Autodesk Inventor part; units mm, degrees
ref_plane "YZ Plane" through (0, 0, 0) normal (1, 0, 0) x (0, 1, 0)
ref_plane "XZ Plane" through (0, 0, 0) normal (0, 1, 0) x (-1, 0, 0)
ref_plane "XY Plane" through (0, 0, 0) normal (0, 0, 1) x (1, 0, 0)
sketch "Эскиз1" plane through (0, 0, 0) normal (0, 0, 1) x (1, 0, 0)
  line L0 (0, 34.036) -> (-10.16, 44.196) construction
  line L1 (0, 0) -> (0, 34.036) construction
  line L2 (-10.16, -10.16) -> (0, 0) construction
  line L3 (-44.196, -10.16) -> (-10.16, -10.16) construction
  line L4 (-54.356, 0) -> (-44.196, -10.16) construction
  line L5 (-54.356, 34.036) -> (-54.356, 0) construction
  line L6 (-44.196, 44.196) -> (-54.356, 34.036) construction
  line L7 (-10.16, 44.196) -> (-44.196, 44.196) construction
  line L8 (1.5, -0.6213) -> (1.5, 34.6573)
  line L9 (1.5, 34.6573) -> (-9.5387, 45.696)
  line L10 (-9.5387, 45.696) -> (-44.8173, 45.696)
  line L11 (-44.8173, 45.696) -> (-55.856, 34.6573)
  line L12 (-55.856, 34.6573) -> (-55.856, -0.6213)
  line L13 (-55.856, -0.6213) -> (-44.8173, -11.66)
  line L14 (-44.8173, -11.66) -> (-9.5387, -11.66)
  line L15 (-9.5387, -11.66) -> (1.5, -0.6213)
  line L16 (-2.7356, -0.7983) -> (-25.2842, -0.7983) construction
  line L17 (-2.7356, 34.7503) -> (-2.7356, -0.7983) construction
  line L18 (-25.2842, 34.7503) -> (-2.7356, 34.7503) construction
  line L19 (-25.2842, -0.7983) -> (-25.2842, 34.7503) construction
  line L20 (-35.7877, 37.522) -> (-26.3913, 37.522) construction
  line L21 (-35.7877, -8.198) -> (-26.3913, -8.198) construction
  line L22 (-26.3913, -0.578) -> (-26.3913, -5.658) construction
  line L23 (-37.7413, -0.578) -> (-37.7413, -5.658) construction
  line L24 (-1.7356, -1.7983) -> (-26.2842, -1.7983)
  line L25 (-26.2842, -1.7983) -> (-26.2842, 35.7503)
  line L26 (-26.2842, 35.7503) -> (-1.7356, 35.7503)
  line L27 (-1.7356, 35.7503) -> (-1.7356, -1.7983)
  line L28 (-26.3913, 37.522) -> (-37.7413, 37.522) construction
  line L29 (-37.7413, 37.522) -> (-37.7413, -8.198) construction
  line L30 (-37.7413, -8.198) -> (-26.3913, -8.198) construction
  line L31 (-26.3913, -8.198) -> (-26.3913, 37.522) construction
  line L32 (-38.2413, 38.022) -> (-25.8913, 38.022)
  line L33 (-25.8913, 38.022) -> (-25.8913, -8.698)
  line L34 (-25.8913, -8.698) -> (-38.2413, -8.698)
  line L35 (-38.2413, -8.698) -> (-38.2413, 38.022)
  point P0 (-25.8913, -1.7983)
  point P1 (-25.8913, 35.7503)
  dimension "d0" = 1.5
  dimension "d1" = 1
  dimension "d2" = 0.5
extrude "Выдавливание1" add sketch "Эскиз1" along normal blind 2
sketch "Эскиз2" plane through (0, 0, 0) normal (0, 0, -1) x (-1, 0, 0)
  line L0 (-1.5, 34.6573) -> (9.5387, 45.696) construction
  line L1 (-1.5, -0.6213) -> (-1.5, 34.6573) construction
  line L2 (9.5387, -11.66) -> (-1.5, -0.6213) construction
  line L3 (44.8173, -11.66) -> (9.5387, -11.66) construction
  line L4 (55.856, -0.6213) -> (44.8173, -11.66) construction
  line L5 (55.856, 34.6573) -> (55.856, -0.6213) construction
  line L6 (44.8173, 45.696) -> (55.856, 34.6573) construction
  line L7 (9.5387, 45.696) -> (44.8173, 45.696) construction
  line L8 (1.7356, 35.7503) -> (1.7356, -1.7983) construction
  line L9 (25.8913, 35.7503) -> (1.7356, 35.7503) construction
  line L10 (25.8913, 38.022) -> (25.8913, 35.7503) construction
  line L11 (38.2413, 38.022) -> (25.8913, 38.022) construction
  line L12 (38.2413, -8.698) -> (38.2413, 38.022) construction
  line L13 (25.8913, -8.698) -> (38.2413, -8.698) construction
  line L14 (25.8913, -1.7983) -> (25.8913, -8.698) construction
  line L15 (1.7356, -1.7983) -> (25.8913, -1.7983) construction
  line L16 (-0.5, 34.2431) -> (9.9529, 44.696)
  line L17 (9.9529, 44.696) -> (44.4031, 44.696)
  line L18 (44.4031, 44.696) -> (54.856, 34.2431)
  line L19 (54.856, 34.2431) -> (54.856, -0.2071)
  line L20 (54.856, -0.2071) -> (44.4031, -10.66)
  line L21 (44.4031, -10.66) -> (9.9529, -10.66)
  line L22 (9.9529, -10.66) -> (-0.5, -0.2071)
  line L23 (-0.5, -0.2071) -> (-0.5, 34.2431)
  line L24 (-1.5, 34.6573) -> (9.5387, 45.696)
  line L25 (9.5387, 45.696) -> (44.8173, 45.696)
  line L26 (44.8173, 45.696) -> (55.856, 34.6573)
  line L27 (55.856, 34.6573) -> (55.856, -0.6213)
  line L28 (55.856, -0.6213) -> (44.8173, -11.66)
  line L29 (44.8173, -11.66) -> (9.5387, -11.66)
  line L30 (9.5387, -11.66) -> (-1.5, -0.6213)
  line L31 (-1.5, -0.6213) -> (-1.5, 34.6573)
  point P0 (0, 0)
  dimension "d0" = 1.5
  dimension "d5" = 1
  dimension "d6" = 1
extrude "Выдавливание2" add sketch "Эскиз2" along normal blind 10
sketch "Эскиз3" plane through (0, 0, 2) normal (0, 0, 1) x (1, 0, 0)
  line L0 (-44.8173, -11.66) -> (-9.5387, -11.66) construction
  line L1 (-9.5387, 45.696) -> (-44.8173, 45.696) construction
  line L2 (-55.856, 34.6573) -> (-55.856, -0.6213) construction
  line L3 (1.5, -0.6213) -> (1.5, 34.6573) construction
  line L4 (-20.178, -11.66) -> (-24.178, -11.66)
  line L5 (-24.178, -11.66) -> (-24.178, -15.66)
  line L6 (-24.178, -15.66) -> (-20.178, -15.66)
  line L7 (-20.178, -15.66) -> (-20.178, -11.66)
  line L8 (-30.178, 45.696) -> (-34.178, 45.696)
  line L9 (-34.178, 45.696) -> (-34.178, 49.696)
  line L10 (-34.178, 49.696) -> (-30.178, 49.696)
  line L11 (-30.178, 49.696) -> (-30.178, 45.696)
  line L12 (1.5, 24.018) -> (5.5, 24.018)
  line L13 (5.5, 24.018) -> (5.5, 20.018)
  line L14 (5.5, 20.018) -> (1.5, 20.018)
  line L15 (1.5, 20.018) -> (1.5, 24.018)
  line L16 (-55.856, 10.018) -> (-59.856, 10.018)
  line L17 (-59.856, 10.018) -> (-59.856, 14.018)
  line L18 (-59.856, 14.018) -> (-55.856, 14.018)
  line L19 (-55.856, 14.018) -> (-55.856, 10.018)
  point P0 (0, 0)
  point P1 (-27.178, -11.66)
  point P2 (1.5, 17.018)
  point P3 (-55.856, 17.018)
  point P4 (-27.178, 45.696)
  dimension "d9" = 4
  dimension "d10" = 4
  dimension "d11" = 3
  dimension "d12" = 4
  dimension "d13" = 4
  dimension "d14" = 4
  dimension "d15" = 4
  dimension "d16" = 4
  dimension "d17" = 4
  dimension "d18" = 3
  dimension "d19" = 3
  dimension "d20" = 3
extrude "Выдавливание3" add sketch "Эскиз3" against normal up to surface (12 mm away)
sketch "Эскиз4" plane through (0, 0, -10) normal (0, 0, -1) x (-1, 0, 0)
  circle A0 centre (-3.5, 22.018) radius 1.5 construction
  circle A1 centre (32.178, 47.696) radius 1.5 construction
  circle A2 centre (57.856, 12.018) radius 1.5 construction
  circle A3 centre (22.178, -13.66) radius 1.5 construction
  circle A4 centre (22.178, -13.66) radius 1
  circle A5 centre (57.856, 12.018) radius 1
  circle A6 centre (32.178, 47.696) radius 1
  circle A7 centre (-3.5, 22.018) radius 1
  point P0 (0, 0)
  dimension "d23" = 2
  dimension "d24" = 2
  dimension "d25" = 2
  dimension "d27" = 2
extrude "Выдавливание4" cut sketch "Эскиз4" against normal through all
properties part number "Низ"
For this review, take the finished solid that the model builds, in its own axes (mm). A direction names the side the tool comes from. Round coordinates to 2 decimals unless told otherwise and drop trailing zeros. Write each loop counter-clockwise with the first axis right and the second up, starting at its lowest first coordinate (ties: lowest second). Pieces come first, ordered by that corner, then holes. Notation, with made-up numbers: M -10.75,55 L 9.25,55 A16 ccw 9.25,69 Z; hole C 2.25,-23 d4. An arc over 180 degrees is marked long. One line per item, written item: value. Start each with the question number.
(1) We need section D-D (y = -13.66). Give the boundary of the cut face in (x, z).
(2) We need section A-A (x = -35.5). Give the boundary of the cut face in (y, z).
(3) We need section C-C (x = 3.5). Give the boundary of the cut face in (y, z).
(4) Wall thickness on line 1 (Y direction, x = -22, z = -5.5); line 2 (X direction, y = 4, z = -7.5); line 3 (Y direction, x = 3.5, z = -6.75): over which ranges is each line inside the solid? List them lowest first.
(5) Machinability: for faces 1 (the flat face through (-14, -1.798, 1)), 2 (the flat face through (-55.856, 24, -4)), 3 (the flat face through (-24.178, -14, -4)), 4 (the flat face through (-49.703, -5.36, -4.93)), which of the approach directions +Z, -Z, +X, -X, +Y, -Y give a long, thin tool a straight path to every point of the face, cutting with its end or side? Answer none if there is none.
(6) We need section B-B (y = 4). Give the boundary of the cut face in (x, z), and give its area (3 significant figures).
(7) The part is to be moulded in two halves that separate along X. For faces 5 (the flat face through (-30.178, 48, -4)), 6 (the cylindrical face through (-58.81, 12.32, -4.08)), 7 (the flat face through (3, 24.018, -4)), say which applies: released by +X, released by -X, zero draft, split by the parting line, or undercut.
(8) Insertion check: pin 1 (1.6 mm diameter, centred on y = -5.5, z = 0.5, fed in from -X); pin 2 (6 mm diameter, centred on y = 21, z = -1.5, fed in from -X); pin 3 (4 mm diameter, centred on y = 5.5, z = -7, fed in from +X). Each pin has a flat end and moves straight along its axis. Give the tip position at first contact, or say it passes through.
Result:
1. outline: M -24.18,-10 L -23.18,-10 L -23.18,2 L -24.18,2 Z; M -21.18,-10 L -20.18,-10 L -20.18,2 L -21.18,2 Z
2. outline: M -11.66,-10 L -10.66,-10 L -10.66,0 L -8.7,0 L -8.7,2 L -11.66,2 Z; M 38.02,0 L 44.7,0 L 44.7,-10 L 45.7,-10 L 45.7,2 L 38.02,2 Z
3. outline: M 20.02,-10 L 21.02,-10 L 21.02,2 L 20.02,2 Z; M 23.02,-10 L 24.02,-10 L 24.02,2 L 23.02,2 Z
4. line 1: -15.66 to -14.64, -12.68 to -10.66, 44.7 to 45.7
4. line 2: -55.86 to -54.86, 0.5 to 1.5
4. line 3: 20.02 to 21.02, 23.02 to 24.02
5. face 1: +Z, -Z
5. face 2: +Z, -Z, -X, +Y
5. face 3: +Z, -Z, -X, -Y
5. face 4: -Z
6. outline: M -55.86,-10 L -54.86,-10 L -54.86,0 L -38.24,0 L -38.24,2 L -55.86,2 Z; M -1.74,0 L 0.5,0 L 0.5,-10 L 1.5,-10 L 1.5,2 L -1.74,2 Z
6. area: 61.7 mm²
7. face 5: released by +X
7. face 6: undercut
7. face 7: zero draft
8. pin 1: x = -51.78
8. pin 2: x = -55.86
8. pin 3: x = 1.5
